Can you work these out from the model? Positions are in its coordinate system, mm. A direction names the side the tool comes from. Round coordinates to 2 decimals unless told otherwise and drop trailing zeros. Write each loop counter-clockwise with the first axis right and the second up, starting at its lowest first coordinate (ties: lowest second). Pieces come first, ordered by that corner, then holes. Notation, with made-up numbers: M 6,58.5 L 15,58.5 A11 ccw 15,78.5 Z; hole C 2,71.25 d11. An arc over 180 degrees is marked long. Use one line per item in the form item = value. Start each with the question number.
```python
from build123d import *

# Parameters (mm, degrees)
CROQUIS1_R              = 4
SALIENTE_EXTRUIR1_DEPTH = 80
CROQUIS1_3_R            = 4
SALIENTE_EXTRUIR2_DEPTH = 7
REDONDEO1_R             = 0.3


with BuildPart() as part:
    # Croquis1 → Saliente-Extruir1 (new body)
    with BuildSketch(Plane.XY):
        Circle(CROQUIS1_R)
    extrude(amount=SALIENTE_EXTRUIR1_DEPTH)

    # Croquis1<3> → Saliente-Extruir2 (add)
    with BuildSketch(Plane.XY):
        Polygon((-4.330127019, -7.5), (4.330127019, -7.5), (8.660254038, 0), (4.330127019, 7.5), (-4.330127019, 7.5), (-8.660254038, 0), align=None)
        Circle(CROQUIS1_3_R, mode=Mode.SUBTRACT)
    extrude(amount=SALIENTE_EXTRUIR2_DEPTH)

    # Redondeo1
    redondeo1_edges = [part.edges().sort_by_distance(p)[0] for p in [
        (-4, 0, 80),
    ]]
    fillet(redondeo1_edges, radius=REDONDEO1_R)


solid = part.part
```
1. Which directions (+Z, -Z, +X, -X, +Y, -Y) give clear straight access to the entire face, cutting with the end or side of a thin tool? Please do faces 1 (the face through (4, 2, 7)), 2 (the face through (0, 0, 80)).
2. Will these pins go through, and if not, where does the flat tip stop? pin 1 (3 mm diameter, centred on x = 0.5, z = 39, fed in from +Y); pin 2 (8 mm diameter, centred on y = 3.5, z = 55.5, fed in from -X); pin 3 (5 mm diameter, centred on y = -0.5, z = 53, fed in from +X); pin 4 (2 mm diameter, centred on x = 6.5, z = 17, fed in from +Y).
3. If we section it at C-C (y = 5): List the corners of the cut face in (x, z) for me.
4. If we section it at B-B (z = 63.5): List the corners of the cut face in (x, y) for me.
5. Please list where these lines run through material, in increasing order: line 1 along Z through (x, y) = (0.5, 6.25); line 2 along X through (y, z) = (-1.5, 50.5).
6. If we section it at A-A (x = 0): List the corners of the cut face in (y, z) for me.
7. If we section it at D-D (x = 7): List the corners of the cut face in (y, z) for me, and give its area (3 significant figures).
Model answer:
q1.face_1 = +Z
q1.face_2 = +Z, +X, -X, +Y, -Y
q2.pin_1 = 4
q2.pin_2 = -4
q2.pin_3 = 4
q2.pin_4 = through
q3.outline = M -5.77,0 L 5.77,0 L 5.77,7 L -5.77,7 Z
q4.outline = C 0,0 d8
q5.line_1 = 0 to 7
q5.line_2 = -3.71 to 3.71
q6.outline = M -7.5,0 L 7.5,0 L 7.5,7 L 4,7 L 4,79.7 A0.3 ccw 3.7,80 L -3.7,80 A0.3 ccw -4,79.7 L -4,7 L -7.5,7 Z
q7.outline = M -2.88,0 L 2.88,0 L 2.88,7 L -2.88,7 Z
q7.area = 40.3 mm2
